from build123d import *

# Parameters (mm, degrees)
SKETCH1_R           = 24
BOSS_EXTRUDE1_DEPTH = 16
SKETCH2_R           = 17.5
BOSS_EXTRUDE2_DEPTH = 10
SKETCH3_R           = 5
CUT_EXTRUDE1_DEPTH  = 26


with BuildPart() as part:
    # Sketch1 → Boss-Extrude1 (new body)
    with BuildSketch(Plane(origin=(0, 0, 0), x_dir=(1, 0, 0), z_dir=(0, 1, 0))):
        Circle(SKETCH1_R)
    extrude(amount=BOSS_EXTRUDE1_DEPTH)

    # Sketch2 → Boss-Extrude2 (add)
    with BuildSketch(Plane(origin=(0, 16, 0), x_dir=(1, 0, 0), z_dir=(0, 1, 0))):
        Circle(SKETCH2_R)
    extrude(amount=BOSS_EXTRUDE2_DEPTH)

    # Sketch3 → Cut-Extrude1 (cut)
    with BuildSketch(Plane(origin=(0, 26, 0), x_dir=(1, 0, 0), z_dir=(0, 1, 0))):
        Circle(SKETCH3_R)
    extrude(amount=-CUT_EXTRUDE1_DEPTH, mode=Mode.SUBTRACT)


solid = part.part
Source: CAD feature listing. Evaluate the final solid. Frame: model axes, mm. A direction names the side the tool comes from. Round coordinates to 2 decimals unless told otherwise and drop trailing zeros. Order: outer loops, then holes, each group sorted by start corner. A loop starts at its lowest first (then second) coordinate and runs counter-clockwise, first axis right, second up. Notation, with made-up numbers: (34, 6.5) -> (71, 6.5) arc R17 ccw to (71, 10.5) -> close; hole circle Ø4 at (39.5, -9). An arc over 180 degrees is marked (long way). Answer as CSV lines item,"result".
Item 1: Section B-B, the plane x = 0. Return loops of the section in (y, z), plus the area to 3 significant figures.
A:
outline,"(0, -24) -> (16, -24) -> (16, -17.5) -> (26, -17.5) -> (26, -5) -> (0, -5) -> close; (0, 5) -> (26, 5) -> (26, 17.5) -> (16, 17.5) -> (16, 24) -> (0, 24) -> close"
area,"858 mm²"
Item 2: Pull-direction query (X, two-part tool) for faces 1 (the face through (-23.977, 7.888, -1.055)), 2 (the face through (-1.08, 13.18, 4.88)), 3 (the face through (0, 0, -6)); classes: pulls with the +X half, pulls with the -X half, needs draft (parallel to the pull), parting line crosses it, or undercut.
A:
face 1,"parting line crosses it"
face 2,"undercut"
face 3,"needs draft"
Item 3: Section A-A, the plane z = 0. Return loops of the section in (x, y).
A:
outline,"(-24, 0) -> (-5, 0) -> (-5, 26) -> (-17.5, 26) -> (-17.5, 16) -> (-24, 16) -> close; (5, 0) -> (24, 0) -> (24, 16) -> (17.5, 16) -> (17.5, 26) -> (5, 26) -> close"
Item 4: Line query: L1, parallel to Z at x = 0, y = 11.5; L2, parallel to Z at x = 0, y = 19. Output: solid intervals per line, ascending.
A:
L1,"-24 to -5, 5 to 24"
L2,"-17.5 to -5, 5 to 17.5"
Item 5: Section D-D, the plane z = 13.5. Return loops of the section in (x, y).
A:
outline,"(-19.84, 0) -> (19.84, 0) -> (19.84, 16) -> (11.14, 16) -> (11.14, 26) -> (-11.14, 26) -> (-11.14, 16) -> (-19.84, 16) -> close"
Item 6: Reachability of faces 4 (the face through (2, 16, 18)), 5 (the face through (4, 26, 4)) from +Z, -Z, +X, -X, +Y, -Y: full face, straight path, thin tool, end or side. Return the list, or none.
A:
face 4,"+Y"
face 5,"+Z, -Z, +X, -X, +Y"
Item 7: Pin query (flat end, axial travel): pin 1 Ø1 at (y, z) = (10, 5.5) entering from +X; pin 2 Ø9 at (x, z) = (0, 0) entering from -Y; pin 3 Ø6 at (x, z) = (-6, 7.5) entering from -Y; pin 4 Ø6 at (x, y) = (10, 23.5) entering from -Z. Return the tip coordinate at first contact, or that it passes through.
A:
pin 1,"x = 23.47"
pin 2,"through"
pin 3,"y = 0"
pin 4,"z = -16.04"
Item 8: Section C-C, the plane y = 9. Return loops of the section in (x, z), plus the area to 3 significant figures.
A:
outline,"circle Ø48 at (0, 0); hole circle Ø10 at (0, 0)"
area,"1,730 mm²"
